```python
from build123d import *

# Parameters (mm, degrees)
PAD002_DEPTH    = 50
SKETCH022_R     = 3.05
SKETCH022_R_2   = 2
POCKET006_DEPTH = 35
FILLET004_R     = 1
CHAMFER005_SIZE = 2


with BuildPart() as part:
    # Sketch021 → Pad002 (new body)
    with BuildSketch(Plane.XZ):
        with BuildLine():
            Line((0, 62), (0, 4))
            ThreePointArc((0, 4), (0.585786, 2.585786), (2, 2))
            Line((2, 2), (28, 2))
            Line((28, 2), (28, 20))
            Line((28, 20), (9, 20))
            ThreePointArc((4, 25), (5.464466, 21.464466), (9, 20))
            Line((4, 25), (4, 62))
            Line((4, 62), (0, 62))
        make_face()
        with BuildLine():
            ThreePointArc((11.5, 15), (6.5, 10), (11.5, 5))
            Line((11.5, 5), (14.5, 5))
            ThreePointArc((14.5, 5), (19.5, 10), (14.5, 15))
            Line((14.5, 15), (11.5, 15))
        make_face(mode=Mode.SUBTRACT)
    extrude(amount=PAD002_DEPTH)

    # Sketch022 → Pocket006 (cut)
    with BuildSketch(Plane.YZ):
        with Locations((-13, 10)):
            Circle(SKETCH022_R)
        with Locations((-38, 50)):
            Circle(SKETCH022_R_2)
        with Locations((-12, 50)):
            Circle(SKETCH022_R_2)
        with Locations((-25, 27.48334)):
            Circle(SKETCH022_R_2)
    extrude(amount=POCKET006_DEPTH, mode=Mode.SUBTRACT)

    # Fillet004
    fillet004_edges = [part.edges().sort_by_distance(p)[0] for p in [
        (4, 0, 43.5),
        (4, -25, 62),
        (4, -50, 43.5),
        (15, 0, 2),
        (18.5, 0, 20),
        (28, 0, 11),
        (18.5, -50, 20),
        (5.464466, -50, 21.464466),
        (5.464466, 0, 21.464466),
        (15, -50, 2),
        (0.585786, -50, 2.585786),
        (0.585786, 0, 2.585786),
        (6.5, 0, 10),
        (19.5, 0, 10),
        (13, 0, 5),
        (13, 0, 15),
        (28, -16.05, 10),
        (6.5, -16.05, 10),
        (6.5, -50, 10),
        (19.5, -50, 10),
        (13, -50, 15),
        (13, -50, 5),
    ]]
    fillet(fillet004_edges, radius=FILLET004_R)

    # Chamfer005
    chamfer005_edges = [part.edges().sort_by_distance(p)[0] for p in [
        (4, -27, 27.48334),
        (4, -40, 50),
        (4, -14, 50),
    ]]
    chamfer(chamfer005_edges, length=CHAMFER005_SIZE)


solid = part.part
```
For this review, take the finished solid that the model builds, in its own axes (mm). A direction names the side the tool comes from. Coordinates: 2 decimals unless noted, no trailing zeros. Write each loop counter-clockwise with the first axis right and the second up, starting at its lowest first coordinate (ties: lowest second). Pieces come first, ordered by that corner, then holes. Notation, with made-up numbers: (46.5, 71) - (100.5, 71) arc R26 ccw to (100.5, 96) - close; hole circle Ø1 at (70.25, 7). An arc over 180 degrees is marked (long way). Answer in a Markdown table with one row per item. Add a question column.
Q1. For P1, Ø3.5, axis at x = 12.5, y = -19, coming from the +Z side; P2, Ø11, axis at y = -36, z = 38, coming from the +X side; P3, Ø6, axis at y = -32, z = 26.5, coming from the +X side, all flat-tipped, find the tip position at first contact; note any pin that passes through.
Q2. Tool access review of faces 5 (the cylindrical face through (19.5, -24.7, 9.9)), 6 (the flat face through (19, -25, 20)), 7 (the flat face through (0, -25, 33)): name each direction out of +Z, -Z, +X, -X, +Y, -Y from which nothing blocks a thin tool from reaching the whole face with its end or side.
Q3. For probe 1 along Z at (x, y) = (22.75, -13); probe 2 along Y at (x, z) = (1.1, 50); probe 3 along Z at (x, y) = (0.7, -12), list the stretches that pass through material, from the lowest coordinate up.
Q4. We need section B-B, the plane z = 36. State the section outline as (x, y) points, and give its area (3 significant figures).
Q5. We need section C-C, the plane y = -13. Count the separate pieces of the cut face and the enclosed holes in it, and give its area (3 significant figures).
Q6. We need section A-A, the plane z = 50. State the section outline as (x, y) points.
Q7. Draft analysis for pull direction Y (two halves, no side actions). For faces 1 (the conical face through (2.125, -10.858, 48.208)), 2 (the flat face through (28, -25, 11)), 3 (the flat face through (11, 0, 17)), 4 (the cylindrical face through (1, -38, 48)), state which applies: +Y half, -Y half, draft (parallel to the pull), parting line (faces both ways), or undercut.
Answer list:
| question | item | result |
|---|---|---|
| 1 | P1 | stops at z = 20 |
| 1 | P2 | stops at x = 4 |
| 1 | P3 | stops at x = 4.23 |
| 2 | face 5 | +Y, -Y |
| 2 | face 6 | +Z, +X, +Y, -Y |
| 2 | face 7 | +Z, -Z, -X, +Y, -Y |
| 3 | probe 1 | z = 2 to 6.95, 13.05 to 20 |
| 3 | probe 2 | y = -50 to -40, -36 to -14, -10 to 0 |
| 3 | probe 3 | z = 2.48 to 7.12, 12.88 to 48, 52 to 62 |
| 4 | outline | (0, -49) arc R1 ccw to (1, -50) - (3, -50) arc R1 ccw to (4, -49) - (4, -1) arc R1 ccw to (3, 0) - (1, 0) arc R1 ccw to (0, -1) - close |
| 4 | area | 199 mm2 |
| 5 | separate pieces | 3 |
| 5 | enclosed holes | 0 |
| 5 | area | 454 mm2 |
| 6 | outline | (0, -49) arc R1 ccw to (1, -50) - (3, -50) arc R1 ccw to (4, -49) - (4, -42) - (2, -40) - (0, -40) - close; (0, -36) - (2, -36) - (4, -34) - (4, -16) - (2, -14) - (0, -14) - close; (0, -10) - (2, -10) - (4, -8) - (4, -1) arc R1 ccw to (3, 0) - (1, 0) arc R1 ccw to (0, -1) - close |
| 7 | face 1 | undercut |
| 7 | face 2 | draft |
| 7 | face 3 | +Y half |
| 7 | face 4 | undercut |
